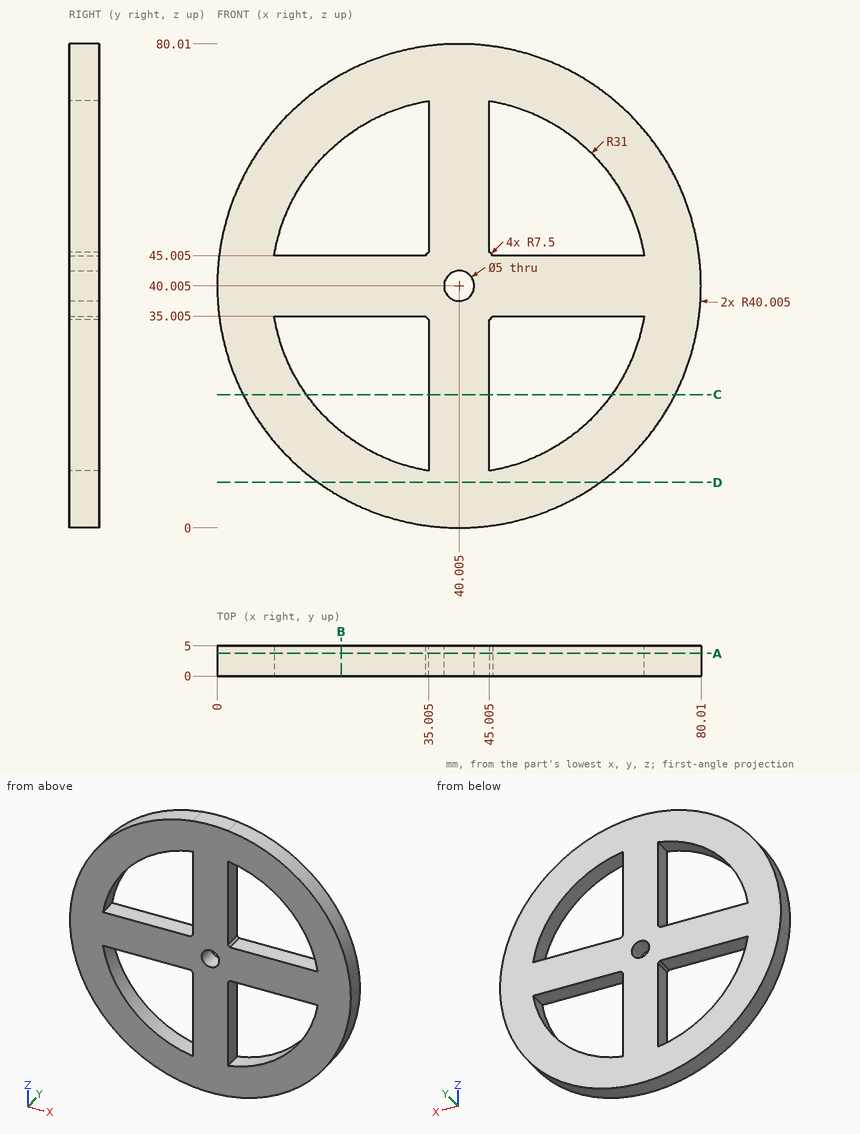
Input: dimensioned drawing with shaded views. Units: mm. Origin: part minimum x, y, z. Round coordinates to 2 decimals unless told otherwise and drop trailing zeros. Loops run counter-clockwise (first coordinate to the right, second up) from the corner with the lowest first, then second, coordinate; pieces in that order, holes last. Notation, with made-up numbers: M 49,-20.75 L 62,-20.75 A16 cw 62,-14.75 Z; hole C 25.25,32 d1. An arc over 180 degrees is marked long. Answer in a Markdown table with one row per item. Add a question column.
1. Contact query for flat-ended pins moving along their axis: pin 1 (1.5 mm diameter, centred on y = 2.5, z = 28, fed in from -X); pin 2 (2 mm diameter, centred on x = 21.5, y = 3.5, fed in from -Z); pin 3 (3 mm diameter, centred on x = 25, y = 3.5, fed in from +Z). Output: stop coordinate, or through.
2. Section A-A (y = 3.75). Output: boundary loops of the cut face in (x, z) (1 decimal), and give its area (3 significant figures).
3. Ray query, probe 1 along Z at (x, y) = (12.5, 1.65) (1 decimal); probe 2 along X at (y, z) = (0.8, 49.5) (3 decimals); probe 3 along X at (y, z) = (2, 13) (1 decimal). Return the intervals inside material, ascending.
4. Section D-D (z = 7.5). Output: boundary loops of the cut face in (x, y) (3 decimals), and give its area (3 significant figures).
5. Section C-C (z = 22). Output: boundary loops of the cut face in (x, y) (1 decimal).
6. Section B-B (x = 20.5). Output: boundary loops of the cut face in (y, z) (1 decimal).
Values follow:
| question | item | result |
|---|---|---|
| 1 | pin 1 | x = 1.62 |
| 1 | pin 2 | z = 4.03 |
| 1 | pin 3 | z = 77.66 |
| 2 | outline | M 0.3,35 A40 ccw 35,0.3 A40 ccw 45,0.3 A40 ccw 79.7,35 A40 ccw 80,40 A40 ccw 79.7,45 A40 ccw 45,79.7 A40 ccw 35,79.7 A40 ccw 0.3,45 A40 ccw Z; hole M 9.4,35 A31 ccw 35,9.4 L 35,34.4 A7.5 cw 34.4,35 Z; hole M 9.4,45 L 34.4,45 A7.5 cw 35,45.6 L 35,70.6 A31 ccw Z; hole C 40,40 d5; hole M 45,9.4 A31 ccw 70.6,35 L 45.6,35 A7.5 cw 45,34.4 Z; hole M 45,45.6 A7.5 cw 45.6,45 L 70.6,45 A31 ccw 45,70.6 Z |
| 2 | area | 3,120 mm^2 |
| 3 | probe 1 | 11 to 25.7, 35 to 45, 54.3 to 69.1 |
| 3 | probe 2 | 1.143 to 10.495, 35.005 to 45.005, 69.515 to 78.867 |
| 3 | probe 3 | 10.5 to 24.8, 35 to 45, 55.2 to 69.5 |
| 4 | outline | M 16.685,0 L 63.325,0 L 63.325,5 L 16.685,5 Z |
| 4 | area | 233 mm^2 |
| 5 | outline | M 4.3,0 L 14.8,0 L 14.8,5 L 4.3,5 Z; M 35,0 L 45,0 L 45,5 L 35,5 Z; M 65.2,0 L 75.7,0 L 75.7,5 L 65.2,5 Z |
| 6 | outline | M 0,5.1 L 5,5.1 L 5,15.9 L 0,15.9 Z; M 0,35 L 5,35 L 5,45 L 0,45 Z; M 0,64.1 L 5,64.1 L 5,74.9 L 0,74.9 Z |
